Could you check a few things on this model? Use its own coordinates, in mm. A direction names the side the tool comes from. Coordinates: 2 decimals unless noted, no trailing zeros. Order: outer loops, then holes, each group sorted by start corner. A loop starts at its lowest first (then second) coordinate and runs counter-clockwise, first axis right, second up. Notation, with made-up numbers: M 49,49 L 55,49 A11 ccw 55,65 Z; hole C 30.25,82 d11. An arc over 180 degrees is marked long. Write item = value, one per line. Start each with the question number.
from build123d import *

# Parameters (mm, degrees)
BOSS_EXTRUDE1_DEPTH = 915
SKETCH2_R           = 20
CUT_EXTRUDE1_DEPTH  = 1000


with BuildPart() as part:
    # Sketch1 → Boss-Extrude1 (new body)
    with BuildSketch(Plane.XY):
        Polygon((-35, 0), (35, 0), (72.087354183, -14.984263737), (71.712747589, -15.911447591), (34.805619691, -1), (-34.805619691, -1), (-71.712747589, -15.911447591), (-72.087354183, -14.984263737), align=None)
    extrude(amount=-BOSS_EXTRUDE1_DEPTH)

    # Sketch2 → Cut-Extrude1 (cut)
    with BuildSketch(Plane(origin=(0, 0, 0), x_dir=(1, 0, 0), z_dir=(0, 1, 0))):
        with Locations(Location((0, 76, 0), (0, 0, 180))):
            Circle(SKETCH2_R)
        with Locations(Location((0, 228, 0), (0, 0, 180))):
            Circle(SKETCH2_R)
        with Locations(Location((0, 380, 0), (0, 0, 180))):
            Circle(SKETCH2_R)
        with Locations(Location((0, 532, 0), (0, 0, 180))):
            Circle(SKETCH2_R)
        with Locations(Location((0, 684, 0), (0, 0, 180))):
            Circle(SKETCH2_R)
        with Locations(Location((0, 836, 0), (0, 0, 180))):
            Circle(SKETCH2_R)
    extrude(amount=-CUT_EXTRUDE1_DEPTH, mode=Mode.SUBTRACT)


solid = part.part
(1) Imagine slicing it at B-B on z = -76. List the corners of the cut face in (x, y) for me, plus the area to 3 significant figures.
(2) Thinking about a two-plate mould opening in Z: for faces 3 (the flat face through (-53, -8.35, -451.1)), 4 (the flat face through (0.3, -0.8, 0)), 5 (the cylindrical face through (2.6, -0.49, -664.17)), which applies, released by +Z, released by -Z, zero draft, split by the parting line, or undercut?
(3) Imagine slicing it at C-C on y = -9. List the corners of the cut face in (x, z) for me, plus the area to 3 significant figures.
(4) Will these pins go through, and if not, where does the flat tip stop? P1, Ø5, axis at y = -4, z = -761, coming from the -X side; P2, Ø3, axis at x = -6.5, z = -339, coming from the -Y side; P3, Ø3, axis at y = -6.5, z = -219, coming from the +X side; P4, Ø24, axis at x = 0, z = -532, coming from the +Y side.
(5) Imagine slicing it at D-D on x = -48. List the corners of the cut face in (y, z) for me, plus the area to 3 significant figures.
(6) For faces 1 (the flat face through (53.284, -7.387, -451.095)), 2 (the flat face through (0, -1, -451)), which set-ups out of +Z, -Z, +X, -X, +Y, -Y let a thin tool reach every point of the face, with its end or its side?
(7) Please list where these lines run through material, in increasing order: probe 1 along Y at (x, z) = (-14, -788); probe 2 along X at (y, z) = (-4, -505.5); probe 3 along X at (y, z) = (-1.5, -461). Write a range as from..to.
(8) Imagine slicing it at A-A on x = 0. List the corners of the cut face in (y, z) for me, plus the area to 3 significant figures.
Response:
q1.outline = M -72.09,-14.98 L -71.71,-15.91 L -34.81,-1 L -20,-1 L -20,0 L -35,0 Z; M 20,-1 L 34.81,-1 L 71.71,-15.91 L 72.09,-14.98 L 35,0 L 20,0 Z
q1.area = 110 mm2
q2.face_3 = zero draft
q2.face_4 = released by +Z
q2.face_5 = undercut
q3.outline = M -57.28,-915 L -54.61,-915 L -54.61,0 L -57.28,0 Z; M 54.61,-915 L 57.28,-915 L 57.28,0 L 54.61,0 Z
q3.area = 4,890 mm2
q4.P1 = -51.09
q4.P2 = -1
q4.P3 = 54.8
q4.P4 = through
q5.outline = M -6.33,-915 L -5.25,-915 L -5.25,0 L -6.33,0 Z
q5.area = 987 mm2
q6.face_1 = +Z, -Z, +X, +Y
q6.face_2 = +Z, -Z, -Y
q7.probe_1 = -1..0
q7.probe_2 = -44.9..-42.23, 42.23..44.9
q7.probe_3 = -38.71..-36.04, 36.04..38.71
q8.outline = M -1,-915 L 0,-915 L 0,-856 L -1,-856 Z; M -1,-816 L 0,-816 L 0,-704 L -1,-704 Z; M -1,-664 L 0,-664 L 0,-552 L -1,-552 Z; M -1,-512 L 0,-512 L 0,-400 L -1,-400 Z; M -1,-360 L 0,-360 L 0,-248 L -1,-248 Z; M -1,-208 L 0,-208 L 0,-96 L -1,-96 Z; M -1,-56 L 0,-56 L 0,0 L -1,0 Z
q8.area = 675 mm2
